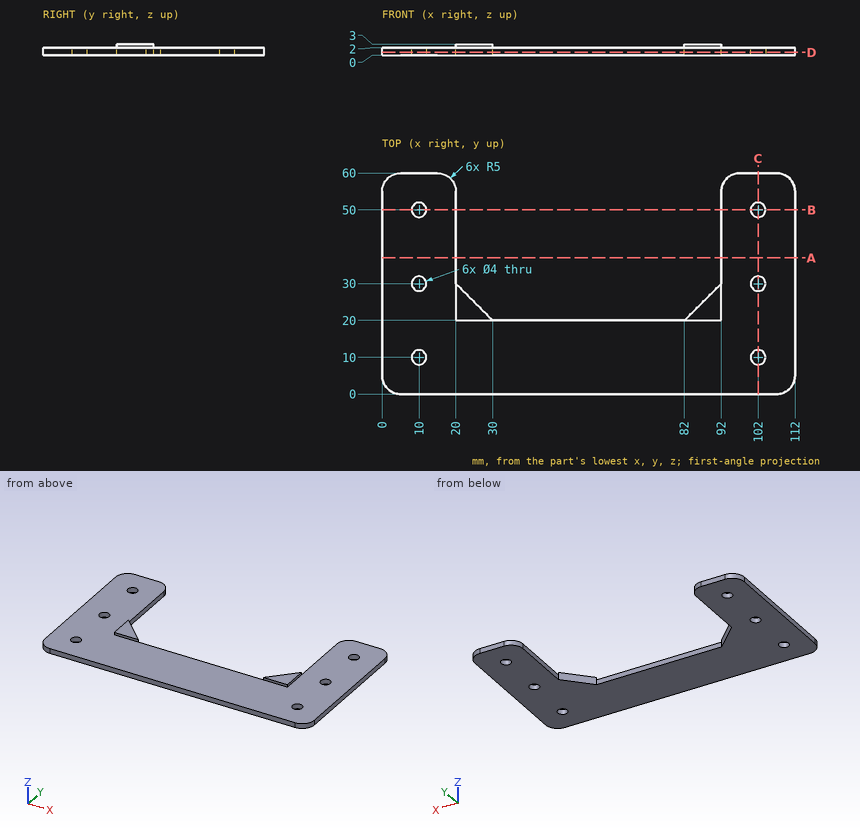
The drawing under review shows one solid part. Ordinate dimensions are in mm from its lowest x, y, z. Coordinates: 2 decimals unless noted, no trailing zeros. Order: outer loops, then holes, each group sorted by start corner. A loop starts at its lowest first (then second) coordinate and runs counter-clockwise, first axis right, second up. Notation, with made-up numbers: M 30.25,-37 L 83.25,-37 A24 ccw 83.25,-24 Z; hole C 50,20 d4. An arc over 180 degrees is marked long. Use a Markdown table: item, result.
(1) Add section C-C (x = 102). Give the boundary of the cut face in (y, z).
Worked answers:
| item | result |
|---|---|
| outline | M 0,0 L 8,0 L 8,2 L 0,2 Z; M 12,0 L 28,0 L 28,2 L 12,2 Z; M 32,0 L 48,0 L 48,2 L 32,2 Z; M 52,0 L 60,0 L 60,2 L 52,2 Z |
(2) Add section D-D (z = 0.7). Give the boundary of the cut face in (x, y), then the cut area to 3 significant figures.
Worked answers:
| item | result |
|---|---|
| outline | M 0,5 A5 ccw 5,0 L 107,0 A5 ccw 112,5 L 112,55 A5 ccw 107,60 L 97,60 A5 ccw 92,55 L 92,30 L 82,20 L 30,20 L 20,30 L 20,55 A5 ccw 15,60 L 5,60 A5 ccw 0,55 Z; hole C 10,10 d4; hole C 10,30 d4; hole C 10,50 d4; hole C 102,10 d4; hole C 102,30 d4; hole C 102,50 d4 |
| area | 3,830 mm2 |
(3) For P1, Ø1.6, axis at x = 54, z = 1, coming from the +Y side; P2, Ø6, axis at x = 22, y = 7, coming from the +Z side; P3, Ø2.5, axis at x = 10, y = 50, coming from the +Z side; P4, Ø0.5, axis at x = 24, z = 2.5, coming from the -Y side, all flat-tipped, find the tip position at first contact; note any pin that passes through.
Worked answers:
| item | result |
|---|---|
| P1 | stops at y = 20 |
| P2 | stops at z = 2 |
| P3 | passes through |
| P4 | stops at y = 20 |
(4) Add section A-A (y = 37). Give the boundary of the cut face in (x, z).
Worked answers:
| item | result |
|---|---|
| outline | M 0,0 L 20,0 L 20,2 L 0,2 Z; M 92,0 L 112,0 L 112,2 L 92,2 Z |
(5) Wall thickness on probe 1 along Y at (x, z) = (102, 1.05); probe 2 along Y at (x, z) = (72, 1.1); probe 3 along Z at (x, y) = (40, 16): over which ranges is each line inside the solid? List them lowest first.
Worked answers:
| item | result |
|---|---|
| probe 1 | y = 0 to 8, 12 to 28, 32 to 48, 52 to 60 |
| probe 2 | y = 0 to 20 |
| probe 3 | z = 0 to 2 |
(6) Add section B-B (y = 50). Give the boundary of the cut face in (x, z), then the cut area to 3 significant figures.
Worked answers:
| item | result |
|---|---|
| outline | M 0,0 L 8,0 L 8,2 L 0,2 Z; M 12,0 L 20,0 L 20,2 L 12,2 Z; M 92,0 L 100,0 L 100,2 L 92,2 Z; M 104,0 L 112,0 L 112,2 L 104,2 Z |
| area | 64.0 mm2 |
